Autodesk Inventor part; units mm, degrees
ref_plane "Work Plane1" through (2.75, 0, 0) normal (0, -1, 0) x (1, 0, 0)
ref_plane "YZ Plane" through (0, 0, 0) normal (1, 0, 0) x (0, 1, 0)
ref_plane "XZ Plane" through (0, 0, 0) normal (0, 1, 0) x (-1, 0, 0)
sketch "Szkic1" plane through (0, 0, 0) normal (0, 0, 1) x (1, 0, 0)
  line L0 (28, 3) -> (28, 0)
  line L1 (-9.5, 0) -> (28, 0)
  line L2 (-17, 0) -> (35.5, 0)
  line L3 (0, 3.6) -> (0, -0.6)
  line L4 (-9.5, 3) -> (-9.5, 0)
  line L5 (10, 3) -> (10, 0) construction
  line L6 (-17, 0) -> (35.5, 0)
  line L7 (-9.5, 3) -> (28, 3)
  dimension "d4" = 9.5
  dimension "d5" = 28
  dimension "d6" = 18
  dimension "d13" = 6
revolve "Bryła" add sketch "Szkic1" angle 360 about axis through (-9.5, 0, 0) along (1, 0, 0)
thread "Gwint1"
thread "Gwint2"
chamfer "Faza1" distance 0.6145 distance2 1 1 edges at (28, -3, 0) measured on face at (28, 1.0659, 1.0214)
chamfer "Faza2" distance 0.6145 distance2 1 1 edges at (-9.5, -3, 0) measured on face at (14.8333, 2.9612, -0.4812)
ref_plane "Work Plane1" through (2.75, 0, 0) normal (0, -1, 0) x (1, 0, 0)
equation "\"d4\" = KOH"
equation "\"d5\" = NLG"
equation "\"d6\" = GEL"
equation "\"d13\" = GD"
equation "\"d1\" = KOH"
equation "\"d7\" = GEL + GAL"
equation "\"d10\" = -0.5 * SPD + 0.5 * GD"
equation "\"d12\" = -0.5 * SPD + 0.5 * GD"
equation "\"NLG\" = 28"
equation "\"GEL\" = 18"
equation "\"GAL\" = 0.61345 * PTC"
equation "\"SPD\" = 4"
equation "\"d0\" = GD"
equation "\"GUL\" = 0.61345 * PTC"
equation "\"KOH\" = 9.5"
equation "\"GD\" = 6"
equation "\"BDM\" = NND"
equation "\"GUL1\" = GUL"
equation "\"GAL1\" = GAL"
equation "\"d80\" = -GUL - GEL"
equation "\"d86\" = -KOH + GUL1"
equation "\"PTC\" = 1"
equation "\"THREADDIA\" = 6"
equation "\"TOA\" = 30deg"
equation "\"NND\" = 6"
equation "\"GD1\" = THREADDIA - 1.2269 * PTC"
properties part number "DIN 835 - M6 x 28" material "Stal, miękka"
The listing builds one solid part. Answer for the finished solid, in the listing's coordinates (mm). Round coordinates to 2 decimals unless told otherwise and drop trailing zeros. Order: outer loops, then holes, each group sorted by start corner. A loop starts at its lowest first (then second) coordinate and runs counter-clockwise, first axis right, second up. Notation, with made-up numbers: (-3.75, 6.25) -> (35.25, 6.25) arc R10 ccw to (35.25, 18.25) -> close; hole circle Ø11 at (76, 77). An arc over 180 degrees is marked (long way). Put each result on its own line as item: value.
Q1. Section A-A, the plane x = 7.5 is taken. Write down the section's boundary in (y, z).
Results list:
outline: circle Ø6 at (0, 0)
Q2. Each of these flat-tipped pins is pushed along its axis until it touches: P1, Ø3, axis at x = 6.5, z = -2, coming from the -Y side; P2, Ø1, axis at y = -2, z = 2, coming from the -X side; P3, Ø1, axis at x = 10, z = 2, coming from the +Y side. Where does it stop, or does it pass through?
Results list:
P1: y = -2.96
P2: x = -9.3
P3: y = 2.6
Q3. Consider line 1 along Y through (x, z) = (16.5, -0.1); line 2 along Y through (x, z) = (-6.5, 1.05). Determine where each line is inside the solid, lowest interval first.
Results list:
line 1: -3 to 3
line 2: -2.81 to 2.81
Q4. Determine the mould class of faces 1 (the flat face through (28, 0, 0)), 2 (the cylindrical face through (9, -3, 0)), 3 (the flat face through (-9.5, 0, 0)) for opening direction X: pulls with the +X half, pulls with the -X half, needs draft (parallel to the pull), parting line crosses it, or undercut.
Results list:
face 1: pulls with the +X half
face 2: needs draft
face 3: pulls with the -X half
